from build123d import *

# Parameters (mm, degrees)
BOSS_EXTRUDE1_DEPTH = 4
BOSS_EXTRUDE2_START = 5
BOSS_EXTRUDE2_DEPTH = 5
BOSS_EXTRUDE3_START = 3
BOSS_EXTRUDE3_DEPTH = 3
CUT_EXTRUDE1_START  = -43
CUT_EXTRUDE1_DEPTH  = 43


with BuildPart() as part:
    # Sketch1 → Boss-Extrude1 (new body)
    with BuildSketch(Plane(origin=(0, 0, 0), x_dir=(1, 0, 0), z_dir=(0, 1, 0))):
        with BuildLine():
            Line((86.216175346, 55.434836598), (79.907674711, 51.378629042))
            ThreePointArc((79.907674711, 51.378629042), (91.148859284, 26.774716641), (95, 0))
            Line((95, 0), (102.5, 0))
            ThreePointArc((102.5, 0), (98.344821859, 28.88851006), (86.216175346, 55.434836598))
        make_face()
        with BuildLine():
            Line((96.730343071, 62.195182525), (90.421842436, 58.138974969))
            ThreePointArc((90.421842436, 58.138974969), (103.142130242, 30.297705673), (107.5, 0))
            Line((107.5, 0), (115, 0))
            ThreePointArc((115, 0), (110.338092817, 32.411499092), (96.730343071, 62.195182525))
        make_face()
        Polygon((102.5, 0), (95, 0), (95, -40), (115, -40), (115, 0), (107.5, 0), (107.5, -20), (102.5, -20), align=None)
    extrude(amount=BOSS_EXTRUDE1_DEPTH)

    # Sketch2 → Boss-Extrude2 (add)
    with BuildSketch(Plane.XZ.offset(BOSS_EXTRUDE2_START)):
        with BuildLine():
            Line((112, 20), (112, 0))
            ThreePointArc((112, 0), (107.459707787, -31.565981725), (94.206942817, -60.572699503))
            Line((94.206942817, -60.572699503), (96.730343071, -62.195182525))
            ThreePointArc((96.730343071, -62.195182525), (110.338092817, -32.411499092), (115, 0))
            Line((115, 0), (115, 20))
            Line((115, 20), (112, 20))
        make_face()
        with BuildLine():
            ThreePointArc((82.431074965, -53.001112065), (94.027244314, -27.620234009), (98, 0))
            Line((98, 0), (98, 20))
            Line((98, 20), (95, 20))
            Line((95, 20), (95, 0))
            ThreePointArc((95, 0), (91.148859284, -26.774716641), (79.907674711, -51.378629042))
            Line((79.907674711, -51.378629042), (82.431074965, -53.001112065))
        make_face()
    extrude(amount=-BOSS_EXTRUDE2_DEPTH)

    # Sketch3 → Boss-Extrude3 (add)
    with BuildSketch(Plane.XZ.offset(5).offset(BOSS_EXTRUDE3_START)):
        with BuildLine():
            Line((98, 20), (112, 20))
            Line((112, 20), (115, 20))
            Line((115, 20), (115, 0))
            ThreePointArc((115, 0), (110.338092817, -32.411499092), (96.730343071, -62.195182525))
            Line((96.730343071, -62.195182525), (94.206942817, -60.572699503))
            Line((94.206942817, -60.572699503), (82.431074965, -53.001112065))
            Line((82.431074965, -53.001112065), (79.907674711, -51.378629042))
            ThreePointArc((79.907674711, -51.378629042), (91.148859284, -26.774716641), (95, 0))
            Line((95, 0), (95, 20))
            Line((95, 20), (98, 20))
        make_face()
    extrude(amount=-BOSS_EXTRUDE3_DEPTH)

    # Sketch4 → Cut-Extrude1 (cut)
    with BuildSketch(Plane(origin=(0, 4, 0), x_dir=(1, 0, 0), z_dir=(0, 1, 0)).offset(CUT_EXTRUDE1_START)):
        with BuildLine():
            Line((90.421842436, 58.138974969), (86.216175346, 55.434836598))
            ThreePointArc((86.216175346, 55.434836598), (98.344821859, 28.88851006), (102.5, 0))
            Line((102.5, 0), (102.5, -20))
            Line((102.5, -20), (107.5, -20))
            Line((107.5, -20), (107.5, 0))
            ThreePointArc((107.5, 0), (103.142130242, 30.297705673), (90.421842436, 58.138974969))
        make_face()
    extrude(amount=CUT_EXTRUDE1_DEPTH, mode=Mode.SUBTRACT)


solid = part.part
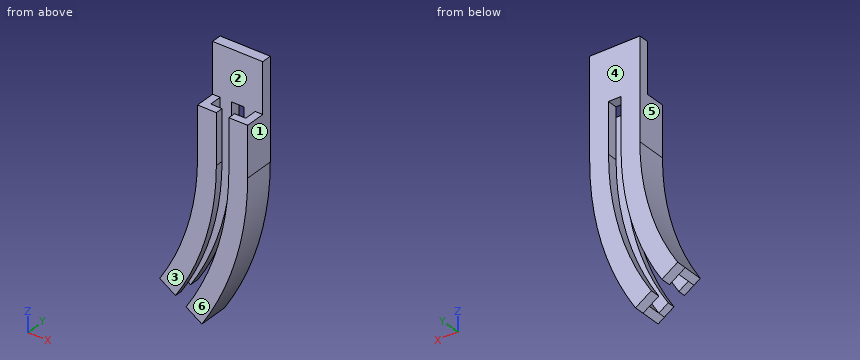
Here's how the part is built. I have some questions about the finished solid (model axes, mm). Face numbers are marked on the shaded views. A direction names the side the tool comes from. Round coordinates to 2 decimals unless told otherwise and drop trailing zeros. Loops run counter-clockwise (first coordinate to the right, second up) from the corner with the lowest first, then second, coordinate; pieces in that order, holes last.
1. If I drill on line 1 along X through (y, z) = (-1, 2); line 2 along Y through (x, z) = (98.5, -47.5); line 3 along X through (y, z) = (3.25, 13.5), over which ranges is the centre line in solid material (lowest first)?
Answer list:
line 1: x = 95 to 98, 112 to 115
line 2: y = -8 to -5, 0 to 4
line 3: x = 95 to 102.5, 107.5 to 115
2. If we section it at B-B on z = -13: Write out the boundary of the cut face in (x, y).
Answer list:
outline: (94.11, -8) - (101.67, -8) - (101.67, -5) - (97.13, -5) - (97.13, 0) - (101.67, 0) - (101.67, 4) - (94.11, 4) - close; (106.71, -8) - (114.26, -8) - (114.26, 4) - (106.71, 4) - (106.71, 0) - (111.24, 0) - (111.24, -5) - (106.71, -5) - close
3. If we section it at C-C on x = 91.5: Write out the boundary of the cut face in (y, z), plus the area to 3 significant figures.
Answer list:
outline: (-8, -58.83) - (-5, -58.83) - (-5, -56.43) - (-8, -56.43) - close; (-8, -46.2) - (-5, -46.2) - (-5, -35.1) - (0, -35.1) - (0, -46.2) - (4, -46.2) - (4, -25.55) - (-8, -25.55) - close; (0, -58.83) - (4, -58.83) - (4, -56.43) - (0, -56.43) - close
area: 209 mm2
4. If we section it at A-A on y = -1.75: Write out the boundary of the cut face in (x, z).
Answer list:
outline: (79.91, -51.38) - (82.43, -53) arc R98 ccw to (98, 0) - (98, 20) - (95, 20) - (95, 0) arc R95 cw to start; (94.21, -60.57) - (96.73, -62.2) arc R115 ccw to (115, 0) - (115, 20) - (112, 20) - (112, 0) arc R112 cw to start
5. For P1, Ø4.5, axis at x = 106, y = 3, coming from the -Z side; P2, Ø2, axis at y = -1, z = -13, coming from the +X side; P3, Ø6, axis at x = 97.5, y = -4.5, coming from the +Z side, each with a flat end and sliding along its axis, tell me the tip position at first contact or that it passes through.
Answer list:
P1: stops at z = -49.61
P2: stops at x = 114.37
P3: stops at z = 20
6. If we section it at D-D on y = -6.75: Write out the boundary of the cut face in (x, z).
Answer list:
outline: (79.91, -51.38) - (86.22, -55.43) arc R102.5 ccw to (102.5, 0) - (102.5, 20) - (95, 20) - (95, 0) arc R95 cw to start; (90.42, -58.14) - (96.73, -62.2) arc R115 ccw to (115, 0) - (115, 20) - (107.5, 20) - (107.5, 0) arc R107.5 cw to start
7. We'd pull the mould along Y, two halves only. Please class the marked faces 1, 2, 3 and 4: +Y half, -Y half, draft (parallel to the pull), parting line (faces both ways), or undercut.
Answer list:
face 1: draft
face 2: undercut
face 3: -Y half
face 4: +Y half
8. Which directions (+Z, -Z, +X, -X, +Y, -Y) give clear straight access to the entire face, cutting with the end or side of a thin tool? Please do the marked faces 5 and 6.
Answer list:
face 5: +Z, -X, +Y, -Y
face 6: +Z, -Z, +X, -X, -Y
